Read the model definition and answer for the solid it produces. Units are mm, in the model's axes. A direction names the side the tool comes from. Round coordinates to 2 decimals unless told otherwise and drop trailing zeros. Write each loop counter-clockwise with the first axis right and the second up, starting at its lowest first coordinate (ties: lowest second). Pieces come first, ordered by that corner, then holes.
from build123d import *

# Parameters (mm, degrees)
ESQUISSE1_W              = 80
ESQUISSE1_H              = 160
BOSS_EXTRU_1_DEPTH       = 5
ESQUISSE2_R              = 1.6
ENL_V_MAT_EXTRU_8_DEPTH  = 10
ESQUISSE3_R              = 1.6
ENL_V_MAT_EXTRU_10_DEPTH = 10
ENL_V_MAT_EXTRU_11_DEPTH = 179.955301682


with BuildPart() as part:
    # Esquisse1 → Boss.-Extru.1 (new body)
    with BuildSketch(Plane(origin=(0, 0, 0), x_dir=(1, 0, 0), z_dir=(0, 1, 0))):
        with Locations((40, 80)):
            Rectangle(ESQUISSE1_W, ESQUISSE1_H)
    extrude(amount=BOSS_EXTRU_1_DEPTH)

    # Esquisse2 → Enlèv. mat.-Extru.8 (cut)
    with BuildSketch(Plane(origin=(0, 0, 0), x_dir=(1, 0, 0), z_dir=(0, 1, 0))):
        with Locations(Location((5, 150, 0), (0, 0, 90))):
            Circle(ESQUISSE2_R)
        with Locations(Location((5, 75, 0), (0, 0, 90))):
            Circle(ESQUISSE2_R)
        with Locations(Location((5, 10, 0), (0, 0, 90))):
            Circle(ESQUISSE2_R)
        with Locations(Location((75, 10, 0), (0, 0, 90))):
            Circle(ESQUISSE2_R)
        with Locations(Location((75, 75, 0), (0, 0, 90))):
            Circle(ESQUISSE2_R)
        with Locations(Location((75, 150, 0), (0, 0, 90))):
            Circle(ESQUISSE2_R)
    extrude(amount=ENL_V_MAT_EXTRU_8_DEPTH, mode=Mode.SUBTRACT)

    # Esquisse3 → Enlèv. mat.-Extru.10 (cut)
    with BuildSketch(Plane(origin=(0, 0, 0), x_dir=(1, 0, 0), z_dir=(0, 1, 0))):
        with Locations(Location((31.225, 8, 0), (0, 0, 90))):
            Circle(ESQUISSE3_R)
        with Locations(Location((48.775, 8, 0), (0, 0, 90))):
            Circle(ESQUISSE3_R)
    extrude(amount=ENL_V_MAT_EXTRU_10_DEPTH, mode=Mode.SUBTRACT)

    # Esquisse4 → Enlèv. mat.-Extru.11 (cut, through all)
    with BuildSketch(Plane(origin=(0, 5, 0), x_dir=(1, 0, 0), z_dir=(0, 1, 0))):
        with BuildLine():
            Line((37.5, 21.5), (42.5, 21.5))
            ThreePointArc((42.5, 21.5), (46, 18), (42.5, 14.5))
            Line((42.5, 14.5), (37.5, 14.5))
            ThreePointArc((37.5, 14.5), (34, 18), (37.5, 21.5))
        make_face()
        with BuildLine():
            Line((30, 50), (50, 50))
            ThreePointArc((50, 50), (55, 45), (50, 40))
            Line((50, 40), (30, 40))
            ThreePointArc((30, 40), (25, 45), (30, 50))
        make_face()
    extrude(amount=-ENL_V_MAT_EXTRU_11_DEPTH, mode=Mode.SUBTRACT)


solid = part.part
Q1. A flat-ended cylindrical pin translates along its axis: pin 1 Ø2.5 at (x, z) = (31.225, -8) entering from -Y. Find the tip coordinate at first contact, or state that the pin passes through.
Verdict:
pin 1: passes through
Q2. Determine the mould class of faces 1 (the flat face through (0, 2, -79)), 2 (the flat face through (80, 2, -79)), 3 (the flat face through (40, 3, -50)), 4 (the flat face through (39, 0, -81)) for opening direction X: pulls with the +X half, pulls with the -X half, needs draft (parallel to the pull), parting line crosses it, or undercut.
Verdict:
face 1: pulls with the -X half
face 2: pulls with the +X half
face 3: undercut
face 4: needs draft
Q3. Section D-D (y = 2.8) is taken. State how many separate pieces and enclosed holes the cut face has, then the cut area to 3 significant figures.
Verdict:
separate pieces: 1
enclosed holes: 10
area: 12,400 mm2
Q4. Which of the six approach directions +Z, -Z, +X, -X, +Y, -Y give full straight-line access (tool end or side, diameter ignored) to faces 5 (the flat face through (40, 3, -21.5)), 6 (the flat face through (39, 2, -160))?
Verdict:
face 5: +Y, -Y
face 6: -Z, +X, -X, +Y, -Y
Q5. Section A-A (x = 5) is taken. Determine the outline of the cut face in (y, z), then the cut area to 3 significant figures.
Verdict:
outline: (0, -160) - (5, -160) - (5, -151.6) - (0, -151.6) - close; (0, -148.4) - (5, -148.4) - (5, -76.6) - (0, -76.6) - close; (0, -73.4) - (5, -73.4) - (5, -11.6) - (0, -11.6) - close; (0, -8.4) - (5, -8.4) - (5, 0) - (0, 0) - close
area: 752 mm2
Q6. Straight lines are drawn through the part: probe 1 along Z at (x, y) = (5, 1.25); probe 2 along X at (y, z) = (1.5, -10); probe 3 along X at (y, z) = (3.15, -18). For each, find the intervals that lie inside material, in ascending order.
Verdict:
probe 1: z = -160 to -151.6, -148.4 to -76.6, -73.4 to -11.6, -8.4 to 0
probe 2: x = 0 to 3.4, 6.6 to 73.4, 76.6 to 80
probe 3: x = 0 to 34, 46 to 80
Q7. Section C-C (z = -75) is taken. Determine the outline of the cut face in (x, y).
Verdict:
outline: (0, 0) - (3.4, 0) - (3.4, 5) - (0, 5) - close; (6.6, 0) - (73.4, 0) - (73.4, 5) - (6.6, 5) - close; (76.6, 0) - (80, 0) - (80, 5) - (76.6, 5) - close
Q8. Section B-B (z = -18) is taken. Determine the outline of the cut face in (x, y).
Verdict:
outline: (0, 0) - (34, 0) - (34, 5) - (0, 5) - close; (46, 0) - (80, 0) - (80, 5) - (46, 5) - close
